Build history of the part. All positions in model axes, mm. Face numbers are marked on the shaded views. Give positions to 0.01 mm unless a question says otherwise; leave off trailing zeros. Order: outer loops, then holes, each group sorted by start corner. A loop starts at its lowest first (then second) coordinate and runs counter-clockwise, first axis right, second up. Notation, with made-up numbers: (-33.5, 5.25) - (4.5, 5.25) arc R27 cw to (4.5, 37.25) - close; hole circle Ø8 at (-13, 16.5). An arc over 180 degrees is marked (long way). Write each question's results on one line, items separated by ' | '. Start each with the question number.
1) Drill centre lines: line 1 along Y through (x, z) = (0, 8.25) (3 decimals); line 2 along Z through (x, y) = (6, 6.25). Where is each one in solid material? Low to high. Write a range as from..to.
2) Drop flat-ended pins along their axis: pin 1 Ø5 at (x, z) = (3.5, 12.5) entering from -Y; pin 2 Ø1.5 at (x, z) = (-7, 39.5) entering from -Y; pin 3 Ø3 at (x, z) = (7.5, 31) entering from +Y; pin 4 Ø1.5 at (x, z) = (-3, 38) entering from +Y. Give the stop position or say it passes through.
3) Cut at B-B on z = 38. List the corners of the cut face in (x, y), plus the area to 3 significant figures.
4) Cut at A-A on z = 22. List the corners of the cut face in (x, y) (3 decimals).
5) Two-plate mould, pull along X, no slides. Class the marked faces 1, 2 and 3: +X half, -X half, draft (parallel to the pull), parting line (faces both ways), or undercut.
from build123d import *

# Parameters (mm, degrees)
F0_R     = 9.525
F1_DEPTH = 50.8
F4_R     = 5.08
F5_R     = 2.794
F6_DEPTH = 13.716
F7_SIZE  = 2.54


with BuildPart() as f1:
    # F0 (on Top) → F1 (new body)
    with BuildSketch(Plane.XY):
        Circle(F0_R)
    extrude(amount=F1_DEPTH)

    # F2 (on Front) → F3 (revolve, cut)
    with BuildSketch(Plane.XZ):
        with BuildLine():
            Line((9.525, 35.7632638335), (9.525, 45.72))
            ThreePointArc((9.525, 45.72), (5.4560644034, 40.7416319168), (9.525, 35.7632638335))
        make_face()
    revolve(axis=Axis((0, 0, -23.9516440779), (0, 0, -1)), mode=Mode.SUBTRACT)

    # F4
    f4_edges = [f1.edges().sort_by_distance(p)[0] for p in [
        (-9.525, 0, 45.72),
        (-9.525, 0, 35.763264),
    ]]
    fillet(f4_edges, radius=F4_R)

    # F5 (on face) → F6 (cut)
    with BuildSketch(Plane(origin=(0, 0, 0), x_dir=(1, 0, 0), z_dir=(0, 0, -1))):
        Circle(F5_R)
    extrude(amount=-F6_DEPTH, mode=Mode.SUBTRACT)

    # F7
    f7_edges = [f1.edges().sort_by_distance(p)[0] for p in [
        (-2.794, 0, 13.716),
    ]]
    chamfer(f7_edges, length=F7_SIZE)


solid = f1.part
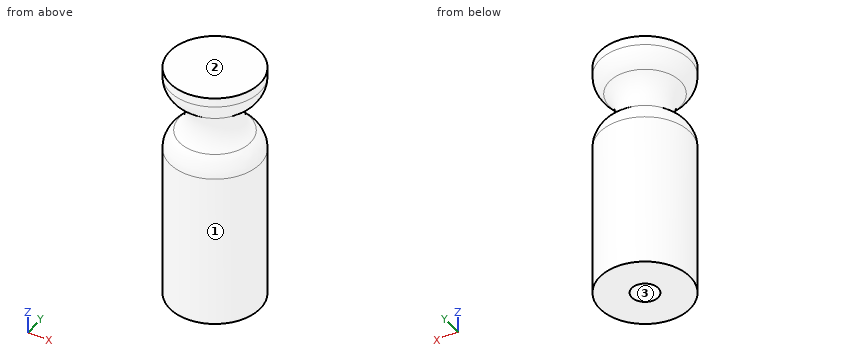
Results:
1) line 1: -9.525..-2.794, 2.794..9.525 | line 2: 0..35.44, 46.04..50.8
2) pin 1: y = -9.47 | pin 2: through | pin 3: y = 7.4 | pin 4: y = 6.23
3) outline: circle Ø12.52 at (0, 0) | area: 123 mm^2
4) outline: circle Ø19.05 at (0, 0)
5) face 1: parting line | face 2: draft | face 3: undercut
